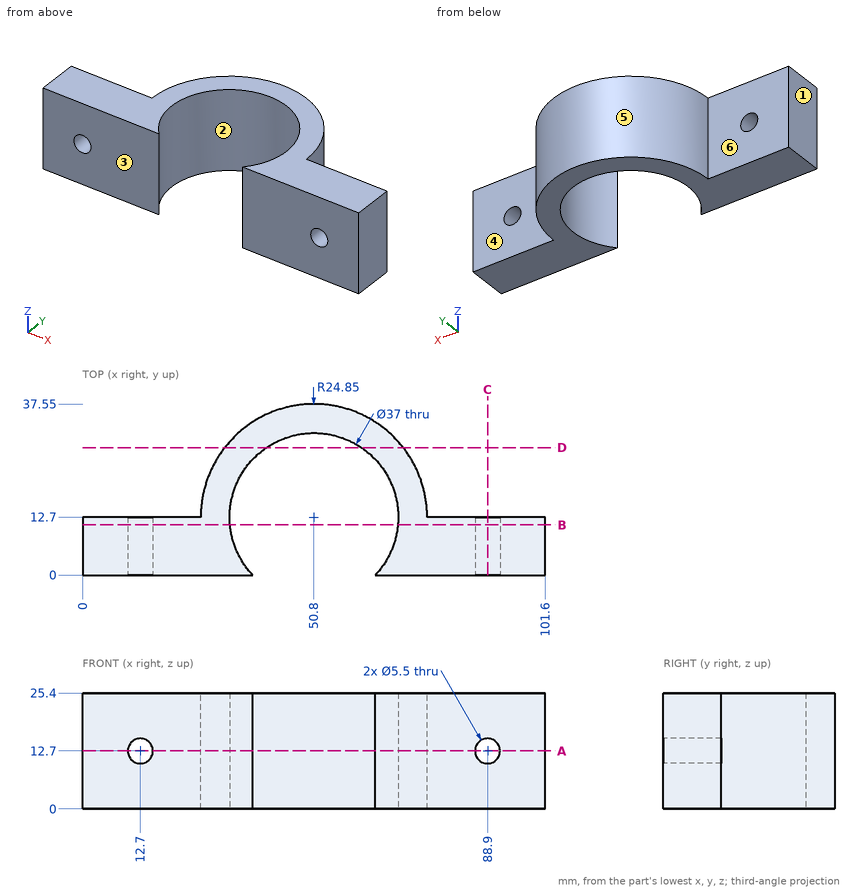
Geometry: see drawing. Coordinates: mm, zero at the bounding-box minimum. A direction names the side the tool comes from. Give positions to 0.01 mm unless a question says otherwise; leave off trailing zeros. Loops run counter-clockwise (first coordinate to the right, second up) from the corner with the lowest first, then second, coordinate; pieces in that order, holes last. Notation, with made-up numbers: (16, -27) -> (42, -27) arc R15 ccw to (42, -23) -> close; hole circle Ø10 at (-14.5, 13). An arc over 180 degrees is marked (long way). Answer as a JSON object with one key per item and string values. Group by question number.
Item 1: Pull-direction query (X, two-part tool) for the marked faces 1, 2 and 3; classes: released by +X, released by -X, zero draft, split by the parting line, or undercut.
Item 2: Cut plane D-D, the plane y = 28. Return the cut outline in (x, z).
Item 3: Cut plane C-C, the plane x = 88.9. Return the cut outline in (y, z).
Item 4: Line query: probe 1 along Z at (x, y) = (12.7, 4.75); probe 2 along X at (y, z) = (7, 12.7); probe 3 along X at (y, z) = (6, 12.7). Output: solid intervals per line, ascending.
Item 5: Cut plane B-B, the plane y = 11. Return the cut outline in (x, z).
Item 6: Reachability of the marked faces 4, 5 and 6 from +Z, -Z, +X, -X, +Y, -Y: full face, straight path, thin tool, end or side. Return the list, or none.
Item 7: Cut plane A-A, the plane z = 12.7. Return the cut outline in (x, y), and give its area (3 significant figures).
Item 8: Pin query (flat end, axial travel): P1, Ø1.5, axis at y = 19.5, z = 20, coming from the +X side; P2, Ø12.5, axis at x = 83, z = 17.5, coming from the +Y side; P3, Ø8, axis at x = 38.5, y = 15.5, coming from the -Z side; P4, Ø6, axis at x = 44.5, z = 20.5, coming from the -Y side. Return the tip coordinate at first contact, or that it passes through.
Checks:
{
 "1": {"face 1": "released by -X", "face 2": "undercut", "face 3": "zero draft"},
 "2": {"outline": "(31.22, 0) -> (40.4, 0) -> (40.4, 25.4) -> (31.22, 25.4) -> close; (61.2, 0) -> (70.38, 0) -> (70.38, 25.4) -> (61.2, 25.4) -> close"},
 "3": {"outline": "(0, 0) -> (12.7, 0) -> (12.7, 9.95) -> (0, 9.95) -> close; (0, 15.45) -> (12.7, 15.45) -> (12.7, 25.4) -> (0, 25.4) -> close"},
 "4": {"probe 1": "z = 0 to 9.95, 15.45 to 25.4", "probe 2": "x = 0 to 9.95, 15.45 to 33.2, 68.4 to 86.15, 91.65 to 101.6", "probe 3": "x = 0 to 9.95, 15.45 to 33.56, 68.04 to 86.15, 91.65 to 101.6"},
 "5": {"outline": "(0, 0) -> (32.38, 0) -> (32.38, 25.4) -> (0, 25.4) -> close; (69.22, 0) -> (101.6, 0) -> (101.6, 25.4) -> (69.22, 25.4) -> close; hole circle Ø5.5 at (12.7, 12.7); hole circle Ø5.5 at (88.9, 12.7)"},
 "6": {"face 4": "+Z, -Z, +X, +Y", "face 5": "+Z, -Z, +Y", "face 6": "+Z, -Z, -X, +Y"},
 "7": {"outline": "(0, 0) -> (9.95, 0) -> (9.95, 12.7) -> (0, 12.7) -> close; (15.45, 0) -> (37.35, 0) arc R18.5 cw (long way) to (64.25, 0) -> (86.15, 0) -> (86.15, 12.7) -> (75.65, 12.7) arc R24.85 ccw to (25.95, 12.7) -> (15.45, 12.7) -> close; (91.65, 0) -> (101.6, 0) -> (101.6, 12.7) -> (91.65, 12.7) -> close", "area": "1,150 mm²"},
 "8": {"P1": "stops at x = 74.9", "P2": "stops at y = 12.7", "P3": "passes through", "P4": "stops at y = 28.69"}
}
